Work out the finished part from the listing and answer in its coordinate system (mm). A direction names the side the tool comes from. Give positions to 0.01 mm unless a question says otherwise; leave off trailing zeros. Write each loop counter-clockwise with the first axis right and the second up, starting at its lowest first coordinate (ties: lowest second). Pieces come first, ordered by that corner, then holes. Notation, with made-up numbers: (28, 15.5) -> (64, 15.5) arc R9 cw to (64, 25.5) -> close; hole circle Ø10 at (21.25, -27). An arc over 180 degrees is marked (long way). Write item = value, one per line. Start each with the question number.
Autodesk Inventor part; units mm, degrees
ref_plane "YZ Plane" through (0, 0, 0) normal (1, 0, 0) x (0, 1, 0)
ref_plane "XZ Plane" through (0, 0, 0) normal (0, 1, 0) x (-1, 0, 0)
ref_plane "XY Plane" through (0, 0, 0) normal (0, 0, 1) x (1, 0, 0)
sketch "Sketch1" plane through (0, 0, 0) normal (0, 1, 0) x (-1, 0, 0)
  line L0 (-18.0542, -22.0034) -> (17.9458, -22.0034)
  line L1 (17.9458, -22.0034) -> (17.9458, 18.9966)
  line L2 (17.9458, 18.9966) -> (-18.0542, 18.9966)
  line L3 (-18.0542, 18.9966) -> (-18.0542, -22.0034)
  line L4 (-18.0542, 18.9966) -> (-0.0043, 18.9966)
  line L5 (-18.0043, 0.0465) -> (-18.0542, 18.9966)
  circle A0 centre (0, 0) radius 11.5
  circle A1 centre (0, 0) radius 12.5
  line L6 (-2.2543, -5.4535) -> (-2.2543, -10.1535)
  line L7 (-2.2543, -10.1535) -> (2.2457, -10.1535)
  line L8 (2.2457, -10.1535) -> (2.2457, -5.4535)
  line L9 (2.2457, -5.4535) -> (-2.2543, -5.4535)
  line L10 (5.9338, 0.7614) -> (9.8309, 3.0114)
  line L11 (9.8309, 3.0114) -> (7.4809, 7.0817)
  line L12 (7.4809, 7.0817) -> (3.5838, 4.8317)
  line L13 (5.9338, 0.7614) -> (3.5838, 4.8317)
  line L14 (-3.5925, 4.8317) -> (-7.4896, 7.0817)
  line L15 (-7.4896, 7.0817) -> (-9.8396, 3.0114)
  line L16 (-9.8396, 3.0114) -> (-5.9425, 0.7614)
  line L17 (-3.5925, 4.8317) -> (-5.9425, 0.7614)
  circle A2 centre (10.1947, -19.139) radius 1.5
  circle A3 centre (-10.3053, 16.611) radius 1.5
  circle A4 centre (10.1947, 16.611) radius 1.5
  circle A5 centre (-10.3053, -19.139) radius 1.5
  line L18 (18.9458, -23.0034) -> (-19.0542, -23.0034)
  line L19 (-19.0542, -23.0034) -> (-19.0542, 19.9966)
  line L20 (-19.0542, 19.9966) -> (18.9458, 19.9966)
  line L21 (18.9458, 19.9966) -> (18.9458, -23.0034)
  line L22 (18.9458, -23.0034) -> (-18.9686, -22.7989) construction
  line L23 (-18.9686, -22.7989) -> (-18.7366, 20.211) construction
  line L24 (-18.7366, 20.211) -> (19.1777, 20.0065) construction
  line L25 (19.1777, 20.0065) -> (18.9458, -23.0034) construction
  point P0 (-0.0043, -1.4535)
  dimension "d0" = 41
  dimension "d1" = 36
  dimension "d2" = 4.7
  dimension "d3" = 4.5
  dimension "d4" = 4.5
  dimension "d5" = 4.7
  dimension "d6" = 3
  dimension "d7" = 3
  dimension "d8" = 3
  dimension "d9" = 3
  dimension "d10" = 1
extrude "Extrusion1" add sketch "Sketch1" against normal blind 1.7 contours L3 L2 L1 L0 | A0 | A1 | L9 L8 L7 L6 | L13 L12 L11 L10 | L17 L16 L15 L14
extrude "Extrusion2" add sketch "Sketch1" along normal blind 2.5 contours L9 L8 L7 L6 | L13 L12 L11 L10 | L17 L16 L15 L14
sketch "Sketch2" plane through (0, -1.7, 0) normal (0, -1, 0) x (1, 0, 0)
  line L0 (18.0542, 18.9966) -> (-17.9458, 18.9966)
  line L1 (8.9542, 19.9966) -> (-8.8458, 19.9966)
  line L2 (-8.8458, 19.9966) -> (-8.8458, 13.9966)
  line L3 (-8.8458, 13.9966) -> (8.9542, 13.9966)
  line L4 (8.9542, 13.9966) -> (8.9542, 19.9966)
  line L5 (18.0542, -22.0034) -> (-17.9458, -22.0034)
  line L6 (0.0542, -22.0034) -> (0.0542, -23.0034)
  line L7 (-8.8458, -23.0034) -> (8.9542, -23.0034)
  line L8 (8.9542, -23.0034) -> (8.9542, -17.0034)
  line L9 (8.9542, -17.0034) -> (-8.8458, -17.0034)
  line L10 (-8.8458, -17.0034) -> (-8.8458, -23.0034)
  point P0 (0, 0)
  dimension "d50" = 17.8
  dimension "d51" = 6
  dimension "d54" = 1
  dimension "d56" = 17.8
  dimension "d57" = 6
extrude "Extrusion3" add sketch "Sketch2" along normal blind 7
properties part number "Spectral_Sensor"
(1) Find the intervals of material crossed by line 1 along Z through (x, y) = (0, -5.75); line 2 along Z through (x, y) = (-9.5, -1.25); line 3 along Y through (x, z) = (7, 12.5), in increasing order.
(2) For faces 1 (the flat face through (2.254, 1, -8)), 2 (the flat face through (7.918, 1.232, 1.902)), 3 (the flat face through (0, 1, -5.454)), 4 (the flat face through (0, -1, -22.003)), determine the directions among +Z, -Z, +X, -X, +Y, -Y from which every point of the face is accessible in a straight line to the end or side of a thin tool.
(3) A cutting plane is placed at D-D, the plane x = -10.5. Write down the section's boundary in (y, z), then the cut area to 3 significant figures.
(4) A cutting plane is placed at A-A, the plane y = -6.5. Write down the section's boundary in (x, z).
(5) Each of these flat-tipped pins is pushed along its axis until it touches: pin 1 (1.8 mm diameter, centred on y = -4.5, z = 17, fed in from +X); pin 2 (1.8 mm diameter, centred on y = -6.5, z = -21, fed in from -X); pin 3 (5 mm diameter, centred on x = -12.5, z = 4.5, fed in from +Y). Where does it stop, or does it pass through?
(6) Determine the mould class of faces 5 (the flat face through (0, -5, 19.997)), 6 (the cylindrical face through (-9.87, -0.838, 15.147)), 7 (the flat face through (4.75, 1.23, 2.83)), 8 (the flat face through (8.648, 1.232, 5.075)) for opening direction X: pulls with the +X half, pulls with the -X half, needs draft (parallel to the pull), parting line crosses it, or undercut.
(7) A cutting plane is placed at C-C, the plane z = -7. Write down the section's boundary in (x, y), then the cut area to 4 significant figures.
(8) A cutting plane is placed at B-B, the plane x = 3. Write down the section's boundary in (y, z), then the cut area to 3 significant figures.
Results list:
q1.line_1 = -23 to -17, 14 to 20
q1.line_2 = -22 to -20.47, -17.81 to 15.28, 17.94 to 19
q1.line_3 = -1.7 to 0
q2.face_1 = +Z, -Z, +X, +Y
q2.face_2 = -Z, +X, +Y
q2.face_3 = +Z, +X, -X, +Y
q2.face_4 = -Z, +X, -X, +Y
q3.outline = (-1.7, -22) -> (0, -22) -> (0, -20.61) -> (-1.7, -20.61) -> close; (-1.7, -17.67) -> (0, -17.67) -> (0, 15.14) -> (-1.7, 15.14) -> close; (-1.7, 18.08) -> (0, 18.08) -> (0, 19) -> (-1.7, 19) -> close
q3.area = 59.7 mm²
q4.outline = (-8.85, -23) -> (8.95, -23) -> (8.95, -17) -> (-8.85, -17) -> close; (-8.85, 14) -> (8.95, 14) -> (8.95, 20) -> (-8.85, 20) -> close
q5.pin_1 = 8.95
q5.pin_2 = -8.85
q5.pin_3 = 0
q6.face_5 = needs draft
q6.face_6 = undercut
q6.face_7 = undercut
q6.face_8 = pulls with the +X half
q7.outline = (-17.95, -1.7) -> (18.05, -1.7) -> (18.05, 0) -> (2.25, 0) -> (2.25, 2.5) -> (-2.25, 2.5) -> (-2.25, 0) -> (-17.95, 0) -> close
q7.area = 72.45 mm²
q8.outline = (-8.7, -23) -> (-1.7, -23) -> (-1.7, -22) -> (0, -22) -> (0, 19) -> (-1.7, 19) -> (-1.7, 20) -> (-8.7, 20) -> (-8.7, 14) -> (-1.7, 14) -> (-1.7, -17) -> (-8.7, -17) -> close
q8.area = 154 mm²
